For this review, take the finished solid that the model builds, in its own axes (mm). A direction names the side the tool comes from. Round coordinates to 2 decimals unless told otherwise and drop trailing zeros. Order: outer loops, then holes, each group sorted by start corner. A loop starts at its lowest first (then second) coordinate and runs counter-clockwise, first axis right, second up. Notation, with made-up numbers: (6.5, 16.25) -> (10.5, 16.25) arc R32 ccw to (10.5, 52.25) -> close; hole circle Ø1 at (8.5, -33). An arc over 180 degrees is marked (long way). Put each result on its own line as item: value. Start each with the question number.
Autodesk Inventor part; units mm, degrees
ref_plane "YZ Plane" through (0, 0, 0) normal (1, 0, 0) x (0, 1, 0)
ref_plane "XZ Plane" through (0, 0, 0) normal (0, 1, 0) x (-1, 0, 0)
ref_plane "XY Plane" through (0, 0, 0) normal (0, 0, 1) x (1, 0, 0)
sketch "Boceto1" plane through (0, 0, 0) normal (0, 1, 0) x (-1, 0, 0)
  line L0 (-100, 87.5) -> (100, 87.5)
  line L1 (100, 87.5) -> (100, -87.5)
  line L2 (100, -87.5) -> (-100, -87.5)
  line L3 (-100, -87.5) -> (-100, 87.5)
  line L4 (-100, 87.5) -> (100, -87.5) construction
  line L5 (100, 87.5) -> (-100, -87.5) construction
  point P0 (0, 0)
  dimension "d0" = 200
  dimension "d1" = 175
extrude "Extrusión1" add sketch "Boceto1" along normal blind 3
fillet "Empalme1" radius 30 2 edges at (-100, 1.5, 87.5) (-100, 1.5, -87.5)
sketch "Boceto2" plane through (0, 3, 0) normal (0, 1, 0) x (1, 0, 0)
  line L0 (100, 87.5) -> (-70, 87.5)
  line L1 (-70, 87.5) -> (5, 87.5)
  line L2 (5, 87.5) -> (5, 68.5)
  line L3 (5, 68.5) -> (-70, 68.5)
  line L4 (-70, 68.5) -> (-70, 87.5)
  point P0 (0, 0)
  dimension "d5" = 75
  dimension "d6" = 19
extrude "Extrusión2" cut sketch "Boceto2" against normal blind 3
mirror "Simetría1" about plane through (0, 0, 0) normal (0, 0, 1) of "Extrusión2"
fillet "Empalme3" radius 5 8 edges at (-70, 1.5, -87.5) (-70, 1.5, -68.5) (5, 1.5, -87.5) (5, 1.5, -68.5) (5, 1.5, 87.5) (5, 1.5, 68.5) (-70, 1.5, 87.5) (-70, 1.5, 68.5)
sketch "Boceto3" plane through (0, 3, 0) normal (0, 1, 0) x (1, 0, 0)
  line L0 (-100, 57.5) -> (-100, -57.5) construction
  line L1 (-100, 0) -> (100, 0) construction
  line L2 (100, -87.5) -> (100, 87.5) construction
  point P0 (0, 0)
  point P1 (80, 15)
  point P2 (60, 15)
  point P3 (80, -15)
  point P4 (60, -15)
  dimension "d11" = 20
  dimension "d12" = 30
  dimension "d13" = 15
  dimension "d14" = 20
hole "Agujero1" at (80, 3, -15) at (60, 3, -15) at (60, 3, 15) at (80, 3, 15) direction (0, -1, 0) diameter 3 end through all
sketch "Boceto5" plane through (0, 3, 0) normal (0, 1, 0) x (1, 0, 0)
  circle A0 centre (60, -15) radius 1.5 construction
  point P0 (0, 0)
  point P1 (70, 0)
  dimension "d22" = 15
  dimension "d23" = 10
hole "Agujero2" at (70, 3, 0) direction (0, -1, 0) diameter 2.5 end through all
sketch "Boceto6" plane through (0, 3, 0) normal (0, 1, 0) x (1, 0, 0)
  line L0 (100, -87.5) -> (100, 87.5) construction
  line L1 (100, 0) -> (-100, 0) construction
  line L2 (-100, 57.5) -> (-100, -57.5) construction
  point P0 (0, 0)
  point P1 (35, 0)
  point P2 (14, 0)
  dimension "d31" = 21
  dimension "d32" = 65
hole "Agujero3" at (35, 3, 0) at (14, 3, 0) direction (0, -1, 0) diameter 3 end through all
sketch "Boceto7" plane through (0, 3, 0) normal (0, 1, 0) x (1, 0, 0)
  line L0 (-90, 66.5) -> (-90, -66.5) construction
  line L1 (15, -77.5) -> (90, -77.5) construction
  line L2 (15, 77.5) -> (90, 77.5) construction
  line L3 (10, -87.5) -> (100, -87.5) construction
  line L4 (100, -87.5) -> (100, 87.5) construction
  line L5 (5, -73.5) -> (5, -82.5) construction
  line L6 (100, 87.5) -> (10, 87.5) construction
  line L7 (-100, 57.5) -> (-100, -57.5) construction
  line L8 (-65, -68.5) -> (0, -68.5) construction
  point P0 (0, 0)
  point P1 (-90, 0)
  dimension "d40" = 10
  dimension "d41" = 10
  dimension "d42" = 10
  dimension "d43" = 10
  dimension "d44" = 10
  dimension "d45" = 2
hole "Agujero4" at (-90, 3, 66.5) at (-90, 3, -66.5) at (90, 3, 77.5) at (90, 3, -77.5) at (15, 3, 77.5) at (15, 3, -77.5) direction (0, -1, 0) diameter 3 depth 8 tip angle 118
sketch "Boceto8" plane through (0, 3, 0) normal (0, 1, 0) x (1, 0, 0)
  line L0 (-100, 57.5) -> (-100, -57.5)
  point P0 (0, 0)
  point P1 (-70, 25)
  point P2 (-18.1608, 8.6361)
  point P3 (-18.1608, -18.8802)
  point P4 (-70, -24.5)
  point P5 (-100, 0)
  dimension "d53" = 49.5
  dimension "d54" = 51.8392
  dimension "d55" = 16.3639
  dimension "d56" = 27.5163
  dimension "d57" = 30
  dimension "d58" = 25
hole "Agujero5" at (-70, 3, -25) at (-18.1608, 3, -8.6361) at (-18.1608, 3, 18.8802) at (-70, 3, 24.5) direction (0, -1, 0) diameter 3 end through all
sketch "Boceto9" plane through (0, 3, 0) normal (0, 1, 0) x (1, 0, 0)
  line L0 (-17, 40) -> (-67, 40)
  line L1 (-67, 40) -> (-67, 35)
  line L2 (-67, 35) -> (-17, 35)
  line L3 (-17, 35) -> (-17, 40)
  line L4 (-100, 57.5) -> (-100, -57.5)
  point P0 (0, 0)
  point P1 (-100, 0)
  dimension "d66" = 5
  dimension "d67" = 33
  dimension "d68" = 50
  dimension "d69" = 35
extrude "Extrusión3" cut sketch "Boceto9" against normal through all
sketch "Boceto10" plane through (0, 3, 0) normal (0, 1, 0) x (1, 0, 0)
  line L0 (-17, -33) -> (-55, -33)
  line L1 (-55, -33) -> (-55, -38)
  line L2 (-55, -38) -> (-17, -38)
  line L3 (-17, -38) -> (-17, -33)
  line L4 (-17, 35) -> (-67, 35) construction
  point P0 (0, 0)
  dimension "d72" = 5
  dimension "d73" = 68
  dimension "d74" = 38
extrude "Extrusión4" cut sketch "Boceto10" against normal through all
sketch "Boceto11" plane through (0, 3, 0) normal (0, 1, 0) x (1, 0, 0)
  line L0 (-100, 57.5) -> (-100, -57.5)
  line L1 (-65, -68.5) -> (0, -68.5)
  point P0 (0, 0)
  point P1 (-65, -48.5)
  dimension "d77" = 35
  dimension "d78" = 20
hole "Agujero6" at (-65, 3, 48.5) direction (0, -1, 0) diameter 4 end through all
properties part number "Base_Superior"
Item 1: For L1, parallel to Z at x = 90, y = 1.35; L2, parallel to Z at x = -52.5, y = 2.4; L3, parallel to Z at x = 70, y = 1.5, list the stretches that pass through material, from the lowest coordinate up.
Item 2: Consider section A-A, the plane x = -41. Write out the cut boundary in (y, z).
Item 3: Consider section B-B, the plane x = -5. Write out the cut boundary in (y, z).
Item 4: Consider section C-C, the plane y = 0.6. Count the separate pieces of the cut face and the enclosed holes in it, plus the area to 3 significant figures.
Item 5: Tool access review of faces 1 (the face through (-93.05, 1.52, -76.7)), 2 (the face through (6.43, 1.48, -86)), 3 (the face through (-68.57, 1.48, 70)): name each direction out of +Z, -Z, +X, -X, +Y, -Y from which nothing blocks a thin tool from reaching the whole face with its end or side.
Item 6: Mouldability with a two-part tool opening along Z and no side actions: class faces 4 (the face through (1, 0, 1)), 5 (the face through (-66.983, 1.479, 48.24)), 6 (the face through (-68.5, 1.48, -69.93)), 7 (the face through (-93.42, 1.52, 76.25)) as +Z half, -Z half, draft (parallel to the pull), parting line (faces both ways), or undercut.
Item 7: Insertion check: pin 1 Ø0.9 at (y, z) = (2, -77) entering from -X; pin 2 Ø0.9 at (x, y) = (-21.5, 2) entering from -Z. Each pin has a flat end and moves straight along its axis. Give the tip position at first contact, or say it passes through.
Evaluation:
1. L1: z = -87.5 to -79, -76 to 76, 79 to 87.5
1. L2: z = -68.5 to -40, -35 to 33, 38 to 68.5
1. L3: z = -87.5 to -1.25, 1.25 to 87.5
2. outline: (0, -68.5) -> (3, -68.5) -> (3, -40) -> (0, -40) -> close; (0, -35) -> (3, -35) -> (3, 33) -> (0, 33) -> close; (0, 38) -> (3, 38) -> (3, 68.5) -> (0, 68.5) -> close
3. outline: (0, -68.5) -> (3, -68.5) -> (3, 68.5) -> (0, 68.5) -> close
4. separate pieces: 1
4. enclosed holes: 20
4. area: 31,200 mm^2
5. face 1: -Z, -X, +Y, -Y
5. face 2: -Z, +Y, -Y
5. face 3: +Z, +Y, -Y
6. face 4: draft
6. face 5: undercut
6. face 6: -Z half
6. face 7: +Z half
7. pin 1: stops at x = -93.18
7. pin 2: stops at z = -68.5
